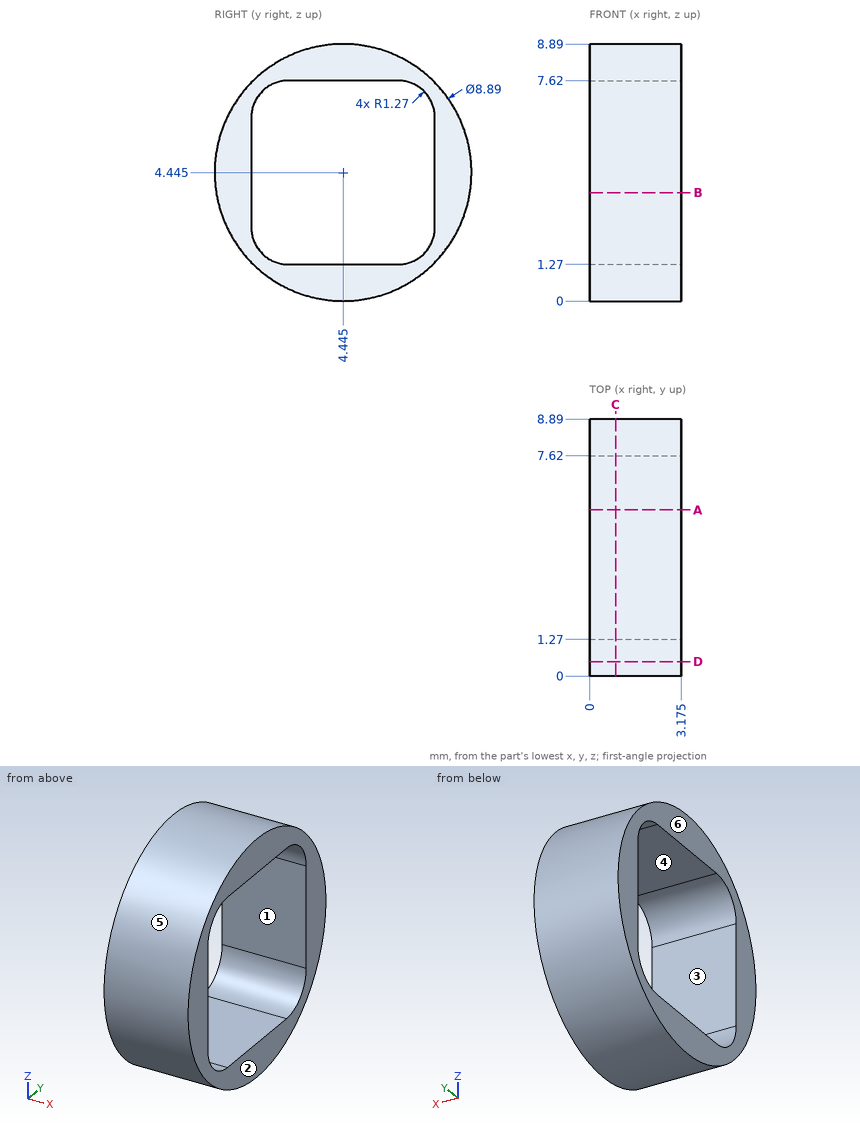
The drawing under review shows one solid part. Ordinate dimensions are in mm from its lowest x, y, z. A direction names the side the tool comes from. Give positions to 0.01 mm unless a question says otherwise; leave off trailing zeros. Order: outer loops, then holes, each group sorted by start corner. A loop starts at its lowest first (then second) coordinate and runs counter-clockwise, first axis right, second up. Notation, with made-up numbers: M 61,3 L 119,3 A32 cw 119,41 Z; hole C 12,-17.5 d1. An arc over 180 degrees is marked long. Answer in a Markdown table with one row per item. Add a question column.
1. Add section C-C on x = 0.9. State the section outline as (y, z) points (3 decimals), plus the area to 3 significant figures.
2. Add section A-A on y = 5.75. State the section outline as (x, z) points (3 decimals), plus the area to 3 significant figures.
3. Machinability: for the marked faces 1 and 2, which of the approach directions +Z, -Z, +X, -X, +Y, -Y give a long, thin tool a straight path to every point of the face, cutting with its end or side? Answer none if there is none.
4. Mouldability with a two-part tool opening along Y and no side actions: class the marked faces 3, 4, 5 and 6 as released by +Y, released by -Y, zero draft, split by the parting line, or undercut.
5. Add section D-D on y = 0.5. State the section outline as (x, z) points (3 decimals), plus the area to 3 significant figures.
6. To check wall thickness, follow line 1 along Y through (x, z) = (0.25, 4.5); line 2 along Z through (x, y) = (0.4, 5.75). State the ranges of each line that lie inside material, in increasing order.
7. Add section B-B on z = 3.75. State the section outline as (x, y) points (3 decimals), plus the area to 3 significant figures.
The answers:
| question | item | result |
|---|---|---|
| 1 | outline | C 4.445,4.445 d8.89; hole M 1.27,2.54 A1.27 ccw 2.54,1.27 L 6.35,1.27 A1.27 ccw 7.62,2.54 L 7.62,6.35 A1.27 ccw 6.35,7.62 L 2.54,7.62 A1.27 ccw 1.27,6.35 Z |
| 1 | area | 23.1 mm2 |
| 2 | outline | M 0,0.196 L 3.175,0.196 L 3.175,1.27 L 0,1.27 Z; M 0,7.62 L 3.175,7.62 L 3.175,8.694 L 0,8.694 Z |
| 2 | area | 6.82 mm2 |
| 3 | face 1 | +X, -X |
| 3 | face 2 | +Z, -Z, +X, +Y, -Y |
| 4 | face 3 | undercut |
| 4 | face 4 | undercut |
| 4 | face 5 | split by the parting line |
| 4 | face 6 | zero draft |
| 5 | outline | M 0,2.397 L 3.175,2.397 L 3.175,6.493 L 0,6.493 Z |
| 5 | area | 13.0 mm2 |
| 6 | line 1 | 0 to 1.27, 7.62 to 8.89 |
| 6 | line 2 | 0.2 to 1.27, 7.62 to 8.69 |
| 7 | outline | M 0,0.055 L 3.175,0.055 L 3.175,1.27 L 0,1.27 Z; M 0,7.62 L 3.175,7.62 L 3.175,8.835 L 0,8.835 Z |
| 7 | area | 7.72 mm2 |
